from build123d import *

# Parameters (mm, degrees)
SKETCH1_W           = 99
SKETCH1_H           = 99
BOSS_EXTRUDE1_DEPTH = 0.5
CUT_EXTRUDE1_DEPTH  = 71.010713466
M2_HOLE1_B_D        = 2.4
M2_HOLE1_B_DEPTH    = 3
M2_HOLE1_B_TIP      = 0.721032743
FILLET1_R           = 0.5


with BuildPart() as part:
    # Sketch1 → Boss-Extrude1 (new, symmetric)
    with BuildSketch(Plane.XY):
        Rectangle(SKETCH1_W, SKETCH1_H)
    extrude(amount=BOSS_EXTRUDE1_DEPTH, both=True)

    # Sketch2 → Cut-Extrude1 (cut, through all)
    with BuildSketch(Plane.XY.offset(0.5)):
        with BuildLine():
            Line((-49.5, 49.5), (-41, 49.5))
            Line((-41, 49.5), (-41, 42.5))
            ThreePointArc((-41, 42.5), (-41.439339828, 41.439339828), (-42.5, 41))
            Line((-42.5, 41), (-49.5, 41))
            Line((-49.5, 41), (-49.5, 49.5))
        make_face()
        with BuildLine():
            Line((49.5, 49.5), (41, 49.5))
            Line((41, 49.5), (41, 42.5))
            ThreePointArc((41, 42.5), (41.439339828, 41.439339828), (42.5, 41))
            Line((42.5, 41), (49.5, 41))
            Line((49.5, 41), (49.5, 49.5))
        make_face()
        with BuildLine():
            Line((-49.5, -49.5), (-41, -49.5))
            Line((-41, -49.5), (-41, -42.5))
            ThreePointArc((-41, -42.5), (-41.439339828, -41.439339828), (-42.5, -41))
            Line((-42.5, -41), (-49.5, -41))
            Line((-49.5, -41), (-49.5, -49.5))
        make_face()
        with BuildLine():
            Line((49.5, -49.5), (41, -49.5))
            Line((41, -49.5), (41, -42.5))
            ThreePointArc((41, -42.5), (41.439339828, -41.439339828), (42.5, -41))
            Line((42.5, -41), (49.5, -41))
            Line((49.5, -41), (49.5, -49.5))
        make_face()
    extrude(amount=-CUT_EXTRUDE1_DEPTH, mode=Mode.SUBTRACT)

    # M2 Hole1 - B
    with Locations(Plane.XY.offset(0.5)):
        with Locations((-45.75, 29), (-29, 45.75), (29, 45.75), (45.75, 29), (45.75, -29), (29, -45.75), (-29, -45.75), (-45.75, -29)):
            Hole(M2_HOLE1_B_D / 2, depth=M2_HOLE1_B_DEPTH)
            with Locations((0, 0, -(M2_HOLE1_B_DEPTH + M2_HOLE1_B_TIP / 2))):  # 118° drill point
                Cone(0, M2_HOLE1_B_D / 2, M2_HOLE1_B_TIP, mode=Mode.SUBTRACT)

    # Fillet1
    fillet1_edges = [part.edges().sort_by_distance(p)[0] for p in [
        (-49.5, 0, 0.5),
        (-46, 41, 0.5),
        (-41.439339828, 41.439339828, 0.5),
        (-41, 46, 0.5),
        (0, 49.5, 0.5),
        (41.439339828, 41.439339828, 0.5),
        (46, 41, 0.5),
        (41, 46, 0.5),
        (49.5, 0, 0.5),
        (41.439339828, -41.439339828, 0.5),
        (41, -46, 0.5),
        (46, -41, 0.5),
        (0, -49.5, 0.5),
        (-41, -46, 0.5),
        (-41.439339828, -41.439339828, 0.5),
        (-46, -41, 0.5),
    ]]
    fillet(fillet1_edges, radius=FILLET1_R)


solid = part.part
Work out the finished part from the listing and answer in its coordinate system (mm). Round coordinates to 2 decimals unless told otherwise and drop trailing zeros. Loops run counter-clockwise (first coordinate to the right, second up) from the corner with the lowest first, then second, coordinate; pieces in that order, holes last. Notation, with made-up numbers: M 83.5,-31.75 L 110.5,-31.75 A34 cw 110.5,5.25 Z; hole C -23,-4 d5. An arc over 180 degrees is marked long. One line per question, with ' | ' between items. Start each with the question number.
(1) Flat-ended cylindrical pins translate along their axes: pin 1 Ø1.4 at (x, y) = (29, 45.75) entering from +Z; pin 2 Ø0.6 at (x, z) = (46.5, -0.5) entering from +Y; pin 3 Ø0.6 at (x, z) = (-47, 0) entering from -Y. Find the tip coordinate at first contact, or state that the pin passes through.
(2) A cutting plane is placed at A-A on z = -0.35. Give the number of separate pieces and of enclosed holes in the cut face, plus the area to 3 significant figures.
(3) A cutting plane is placed at C-C on y = -45.75. Write down the section's boundary in (x, z).
(4) For a pull along Y with two mould halves and no side action, classify faces 1 (the face through (-46.86, 28.54, -0.01)), 2 (the face through (-1, 1, -0.5)) as released by +Y, released by -Y, zero draft, split by the parting line, or undercut.
(5) A cutting plane is placed at B-B on y = 29. Write down the section's boundary in (x, z), plus the area to 3 significant figures.
(6) Find the intervals of material crossed by line 1 (Y direction, x = 29, z = -0.1); line 2 (Y direction, x = -45.75, z = 0); line 3 (Y direction, x = -42.5, z = 0), in increasing order.
Geometry check:
1) pin 1: passes through | pin 2: stops at y = 41 | pin 3: stops at y = -41
2) separate pieces: 1 | enclosed holes: 8 | area: 9,480 mm²
3) outline: M -41,-0.5 L -30.2,-0.5 L -30.2,0.5 L -40.5,0.5 A0.5 ccw -41,0 Z; M -27.8,-0.5 L 27.8,-0.5 L 27.8,0.5 L -27.8,0.5 Z; M 30.2,-0.5 L 41,-0.5 L 41,0 A0.5 ccw 40.5,0.5 L 30.2,0.5 Z
4) face 1: undercut | face 2: zero draft
5) outline: M -49.5,-0.5 L -46.95,-0.5 L -46.95,0.5 L -49,0.5 A0.5 ccw -49.5,0 Z; M -44.55,-0.5 L 44.55,-0.5 L 44.55,0.5 L -44.55,0.5 Z; M 46.95,-0.5 L 49.5,-0.5 L 49.5,0 A0.5 ccw 49,0.5 L 46.95,0.5 Z | area: 94.1 mm²
6) line 1: y = -49.5 to -46.95, -44.55 to 44.55, 46.95 to 49.5 | line 2: y = -41 to -30.2, -27.8 to 27.8, 30.2 to 41 | line 3: y = -41 to 41
